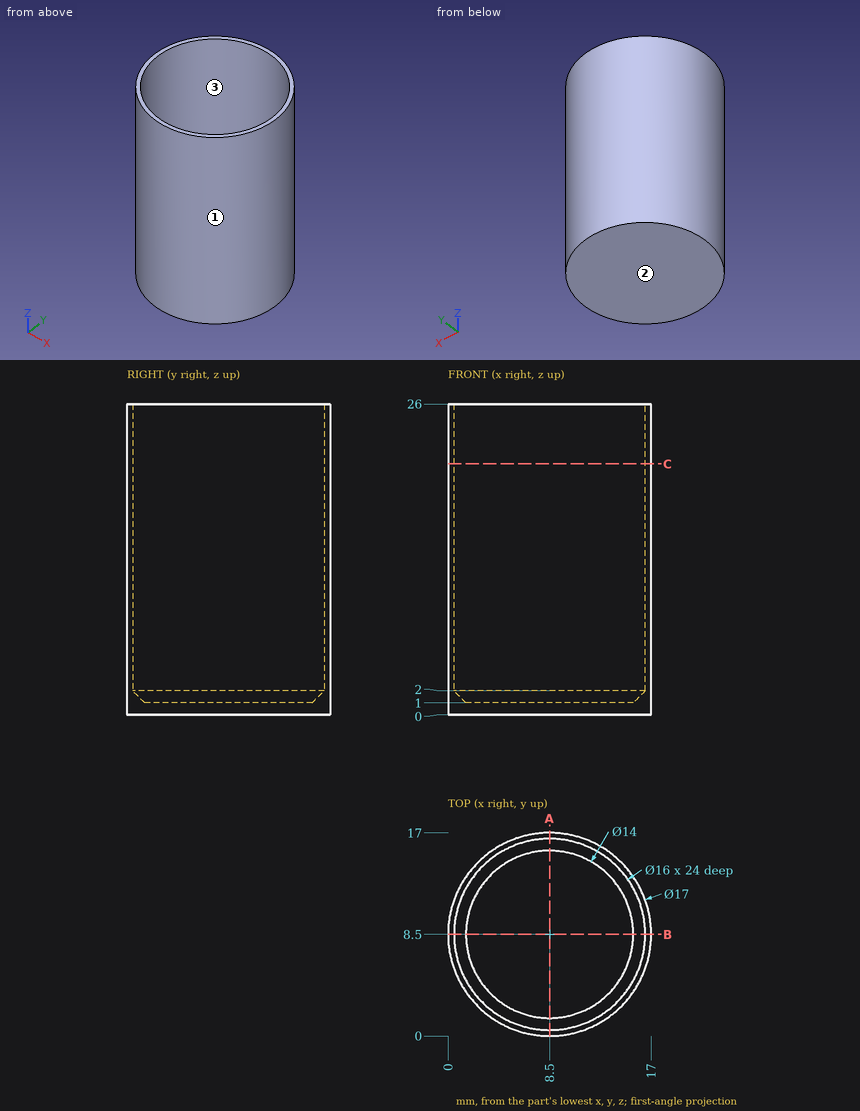
Answer from the drawing. Dimensions are ordinates in mm from the lowest x, y and z of the part. Give positions to 0.01 mm unless a question says otherwise; leave off trailing zeros. Write each loop counter-clockwise with the first axis right and the second up, starting at its lowest first coordinate (ties: lowest second). Pieces come first, ordered by that corner, then holes. Notation, with made-up numbers: (47.5, 81.5) - (77.5, 81.5) arc R12 cw to (77.5, 102.5) - close; hole circle Ø9 at (11.25, -37.5). An arc over 180 degrees is marked (long way). Answer in a Markdown table with one row per item. Add a question column.
Item 1: Determine the mould class of the marked faces 1, 2 and 3 for opening direction Y: pulls with the +Y half, pulls with the -Y half, needs draft (parallel to the pull), parting line crosses it, or undercut.
Item 2: Section A-A, the plane x = 8.5 is taken. Write down the section's boundary in (y, z), and give its area (3 significant figures).
Item 3: Flat-ended cylindrical pins translate along their axes: P1, Ø1.5, axis at y = 6, z = 8.5, coming from the +X side; P2, Ø1.5, axis at x = 7, z = 6.5, coming from the +Y side; P3, Ø2, axis at x = 15, z = 9, coming from the -Y side. Find the tip coordinate at first contact, or state that the pin passes through.
Item 4: Section C-C, the plane z = 21 is taken. Write down the section's boundary in (x, y).
Item 5: Find the intervals of material crossed by L1, parallel to Y at x = 8.5, z = 14; L2, parallel to Z at x = 8.5, y = 11.75; L3, parallel to Y at x = 4, z = 19, in increasing order.
Recorded:
| question | item | result |
|---|---|---|
| 1 | face 1 | parting line crosses it |
| 1 | face 2 | needs draft |
| 1 | face 3 | undercut |
| 2 | outline | (0, 0) - (17, 0) - (17, 26) - (16.5, 26) - (16.5, 2) - (15.5, 1) - (1.5, 1) - (0.5, 2) - (0.5, 26) - (0, 26) - close |
| 2 | area | 43.0 mm2 |
| 3 | P1 | stops at x = 16.82 |
| 3 | P2 | stops at y = 16.97 |
| 3 | P3 | stops at y = 2.02 |
| 4 | outline | circle Ø17 at (8.5, 8.5); hole circle Ø16 at (8.5, 8.5) |
| 5 | L1 | y = 0 to 0.5, 16.5 to 17 |
| 5 | L2 | z = 0 to 1 |
| 5 | L3 | y = 1.29 to 1.89, 15.11 to 15.71 |
